Can you work these out from the model? Positions are in its coordinate system, mm. Face numbers are marked on the shaded views. A direction names the side the tool comes from. Give positions to 0.01 mm unless a question says otherwise; leave off trailing zeros. Loops run counter-clockwise (first coordinate to the right, second up) from the corner with the lowest first, then second, coordinate; pieces in that order, holes last. Notation, with made-up numbers: (54, 29.25) - (111, 29.25) arc R23 cw to (111, 52.25) - close; hole circle Ø11 at (-35.75, 68). An arc over 180 degrees is marked (long way). Answer as a JSON object with one key per item and string values. Group by question number.
Item 1: Please list where these lines run through material, in increasing order: L1, parallel to Y at x = 3.15, z = 29.5; L2, parallel to X at y = -15, z = -19; L3, parallel to Z at x = 26.5, y = -11.
Item 2: Suppose I cut it at A-A on z = 19.5. Write out the boundary of the cut face in (x, y).
Item 3: Which directions (+Z, -Z, +X, -X, +Y, -Y) give clear straight access to the entire face, cutting with the end or side of a thin tool? Please do the marked faces 1, 2 and 3.
Item 4: Suppose I cut it at C-C on z = -19.5. Write out the boundary of the cut face in (x, y), and give its area (3 significant figures).
Item 5: Suppose I cut it at D-D on y = 4. Write out the boundary of the cut face in (x, z).
Item 6: Will these pins go through, and if not, where does the flat tip stop? pin 1 (6.5 mm diameter, centred on x = 24, z = 10.5, fed in from +Y); pin 2 (8 mm diameter, centred on y = -7.5, z = -9.5, fed in from -X); pin 3 (2.5 mm diameter, centred on x = 14, y = -13.5, fed in from -Z); pin 4 (8.5 mm diameter, centred on x = 16.5, y = 8.5, fed in from -Z).
Item 7: Suppose I cut it at B-B on x = 30. Write out the boundary of the cut face in (y, z), and give its area (3 significant figures).
from build123d import *

# Parameters (mm, degrees)
SKETCH1_W           = 69
SKETCH1_H           = 34
SKETCH1_R           = 1.3
SKETCH1_R_2         = 10
BOSS_EXTRUDE1_DEPTH = 5
SKETCH2_W           = 49
SKETCH2_H           = 5
BOSS_EXTRUDE2_DEPTH = 30
BOSS_EXTRUDE3_DEPTH = 2.5
SKETCH4_R           = 1.55
CUT_EXTRUDE1_DEPTH  = 5


with BuildPart() as part:
    # Sketch1 → Boss-Extrude1 (new body)
    with BuildSketch(Plane(origin=(0, 0, 0), x_dir=(0, 0, -1), z_dir=(1, 0, 0))):
        Rectangle(SKETCH1_W, SKETCH1_H)
        with Locations((-29.5, 12)):
            Circle(SKETCH1_R, mode=Mode.SUBTRACT)
        with Locations((-29.5, -12)):
            Circle(SKETCH1_R, mode=Mode.SUBTRACT)
        with Locations((29.5, 12)):
            Circle(SKETCH1_R, mode=Mode.SUBTRACT)
        with Locations((29.5, -12)):
            Circle(SKETCH1_R, mode=Mode.SUBTRACT)
        with Locations((19.5, 0)):
            Circle(SKETCH1_R_2, mode=Mode.SUBTRACT)
    extrude(amount=BOSS_EXTRUDE1_DEPTH)

    # Sketch2 → Boss-Extrude2 (add)
    with BuildSketch(Plane(origin=(5, 0, 0), x_dir=(0, 0, -1), z_dir=(1, 0, 0))):
        with Locations((0, -14.5)):
            Rectangle(SKETCH2_W, SKETCH2_H)
    extrude(amount=BOSS_EXTRUDE2_DEPTH)

    # Sketch3 → Boss-Extrude3 (add, symmetric)
    with BuildSketch(Plane.XY):
        Polygon((5, -12), (35, -12), (5, 17), align=None)
    extrude(amount=BOSS_EXTRUDE3_DEPTH, both=True)

    # Sketch4 → Cut-Extrude1 (cut)
    with BuildSketch(Plane.XZ.offset(17)):
        with Locations(Location((30, 19.5, 0), (0, 0, 270))):
            Circle(SKETCH4_R)
        with Locations(Location((10, 19.5, 0), (0, 0, 270))):
            Circle(SKETCH4_R)
        with Locations(Location((10, -19.5, 0), (0, 0, 90))):
            Circle(SKETCH4_R)
        with Locations(Location((30, -19.5, 0), (0, 0, 90))):
            Circle(SKETCH4_R)
    extrude(amount=-CUT_EXTRUDE1_DEPTH, mode=Mode.SUBTRACT)


solid = part.part
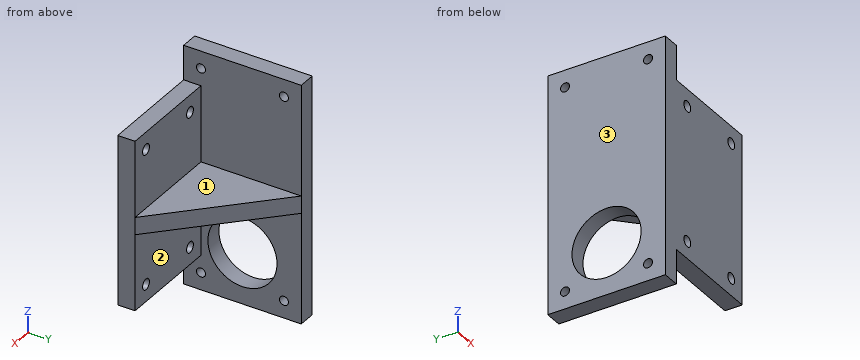
Worked out:
{
 "1": {"L1": "y = -17 to -13.3, -10.7 to 10.7, 13.3 to 17", "L2": "x = 0 to 8.53, 11.47 to 28.53, 31.47 to 35", "L3": "z = -2.5 to 2.5"},
 "2": {"outline": "(0, -17) - (8.45, -17) - (8.45, -12) - (5, -12) - (5, 17) - (0, 17) - close; (11.55, -17) - (28.45, -17) - (28.45, -12) - (11.55, -12) - close; (31.55, -17) - (35, -17) - (35, -12) - (31.55, -12) - close"},
 "3": {"face 1": "+Z, +X, +Y", "face 2": "-Z, +X, +Y", "face 3": "+Z, -Z, -X, +Y, -Y"},
 "4": {"outline": "(0, -17) - (8.45, -17) - (8.45, -12) - (5, -12) - (5, -10) - (0, -10) - close; (0, 10) - (5, 10) - (5, 17) - (0, 17) - close; (11.55, -17) - (28.45, -17) - (28.45, -12) - (11.55, -12) - close; (31.55, -17) - (35, -17) - (35, -12) - (31.55, -12) - close", "area": "189 mm2"},
 "5": {"outline": "(0, -34.5) - (5, -34.5) - (5, -28.67) - (0, -28.67) - close; (0, -10.33) - (5, -10.33) - (5, -2.5) - (18.45, -2.5) - (18.45, 2.5) - (5, 2.5) - (5, 34.5) - (0, 34.5) - close"},
 "6": {"pin 1": "stops at y = -12", "pin 2": "stops at x = 0", "pin 3": "stops at z = -24.5", "pin 4": "stops at z = -2.5"},
 "7": {"outline": "(-17, -24.5) - (-12, -24.5) - (-12, -21.05) - (-17, -21.05) - close; (-17, -17.95) - (-12, -17.95) - (-12, -2.5) - (-7.17, -2.5) - (-7.17, 2.5) - (-12, 2.5) - (-12, 17.95) - (-17, 17.95) - close; (-17, 21.05) - (-12, 21.05) - (-12, 24.5) - (-17, 24.5) - close", "area": "238 mm2"}
}
